from build123d import *

# Parameters (mm, degrees)
F1_DEPTH = 25
F0_W     = 5
F0_H     = 35.8
F2_DEPTH = 2.5


with BuildPart() as f1:
    # F0 (on Front) → F1 (new body, symmetric)
    with BuildSketch(Plane.XZ):
        Polygon((20, 0), (-25, 0), (-25, -10), (25, -10), (25, 0), align=None)
    extrude(amount=F1_DEPTH, both=True)

    # F0 (on Front) → F2 (join, symmetric)
    with BuildSketch(Plane.XZ):
        with Locations((22.5, 17.9)):
            Rectangle(F0_W, F0_H)
        Polygon((19, 35.8), (20, 35.8), (25, 35.8), (25, 40.8), (20, 40.8), align=None)
        Polygon((0, 35.8), (19, 35.8), (20, 40.8), (0, 40.8), align=None)
    extrude(amount=F2_DEPTH, both=True)

    # F0 (on Front) → F3 (revolve)
    with BuildSketch(Plane.XZ):
        Polygon((12, 0.8), (19, 35.8), (0, 35.8), (0, 0.8), align=None)
        Polygon((0, 35.8), (19, 35.8), (20, 40.8), (0, 40.8), align=None)
    revolve(axis=Axis((0, 0, 20.8), (0, 0, -1)))


solid = f1.part
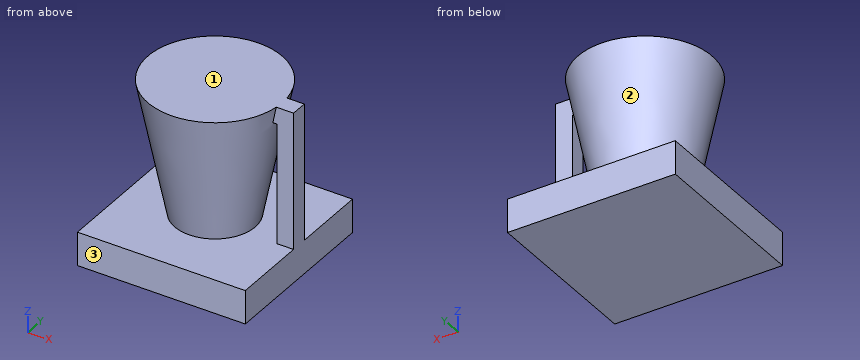
Geometry check sheet. Reference: the model listing, model coordinates, mm. Face numbers are marked on the shaded views. Give positions to 0.01 mm unless a question says otherwise; leave off trailing zeros. Order: outer loops, then holes, each group sorted by start corner. A loop starts at its lowest first (then second) coordinate and runs counter-clockwise, first axis right, second up.
1) Cross-section at A-A (z = 27). Record the boundary of the cut face in (x, y).
Results are:
outline: circle Ø34.48 at (0, 0); (20, -2.5) - (25, -2.5) - (25, 2.5) - (20, 2.5) - close
2) Cross-section at C-C (y = 0). Record the boundary of the cut face in (x, z), then the cut area to 3 significant figures.
Results are:
outline: (-25, -10) - (25, -10) - (25, 40.8) - (-20, 40.8) - (-12, 0.8) - (12, 0.8) - (19, 35.8) - (20, 35.8) - (20, 0) - (-25, 0) - close
area: 1,990 mm2
3) Cross-section at B-B (x = 0). Record the boundary of the cut face in (y, z), then the cut area to 3 significant figures.
Results are:
outline: (-25, -10) - (25, -10) - (25, 0) - (-25, 0) - close; (-20, 40.8) - (-12, 0.8) - (12, 0.8) - (20, 40.8) - close
area: 1,780 mm2
4) Cross-section at D-D (z = 2). Record the boundary of the cut face in (x, y).
Results are:
outline: circle Ø24.48 at (0, 0); (20, -2.5) - (25, -2.5) - (25, 2.5) - (20, 2.5) - close
5) Material ranges on probe 1 along Z at (x, y) = (-5.5, -9); probe 2 along Z at (x, y) = (4, -21); probe 3 along X at (y, z) = (-2, 4), recorded low to high.
Results are:
probe 1: z = -10 to 0, 0.8 to 40.8
probe 2: z = -10 to 0
probe 3: x = -12.48 to 12.48, 20 to 25
6) Gauge pin test, flat ends, axial feed: pin 1 (4 mm diameter, centred on y = -1, z = 25, fed in from -X); pin 2 (7 mm diameter, centred on x = 22, z = 30, fed in from +Y); pin 3 (6 mm diameter, centred on x = -3, z = 28, fed in from +Y). Record the tip position at first contact, or that the pin passes through.
Results are:
pin 1: stops at x = -17.22
pin 2: stops at y = 2.5
pin 3: stops at y = 17.9
7) Draft check along Z on the marked faces 1, 2 and 3. Enter one of: released by +Z, released by -Z, zero draft, split by the parting line, or undercut.
Results are:
face 1: released by +Z
face 2: undercut
face 3: zero draft
